Verification items for the finished model (mm, model axes). Round coordinates to 2 decimals unless told otherwise and drop trailing zeros. Write each loop counter-clockwise with the first axis right and the second up, starting at its lowest first coordinate (ties: lowest second). Pieces come first, ordered by that corner, then holes. Notation, with made-up numbers: M -33,82.5 L -10,82.5 A10 cw -10,86.5 Z; hole C 58.5,7.25 d5. An arc over 180 degrees is marked long. One line per question, with ' | ' between items. Start each with the question number.
Q1. Gauge pin test, flat ends, axial feed: pin 1 (4 mm diameter, centred on x = -49.5, z = -42.5, fed in from +Y); pin 2 (6.5 mm diameter, centred on x = -40, y = -33, fed in from -Z); pin 3 (3 mm diameter, centred on y = -12.5, z = -19, fed in from +X); pin 4 (8 mm diameter, centred on x = -29, y = -33.5, fed in from +Z). Record the tip position at first contact, or that the pin passes through.
Q2. Thickness scan on line 1 along Y through (x, z) = (-31, -17); line 2 along Y through (x, z) = (-51, -50); line 3 along X through (y, z) = (-3, -46.5). Record the ranges inside material, lowest first. Write a range as from..to.
Q3. Cross-section at B-B (z = -6). Record the boundary of the cut face in (x, y), then the cut area to 3 significant figures.
Q4. Cross-section at A-A (x = -56.5). Record the boundary of the cut face in (y, z), then the cut area to 3 significant figures.
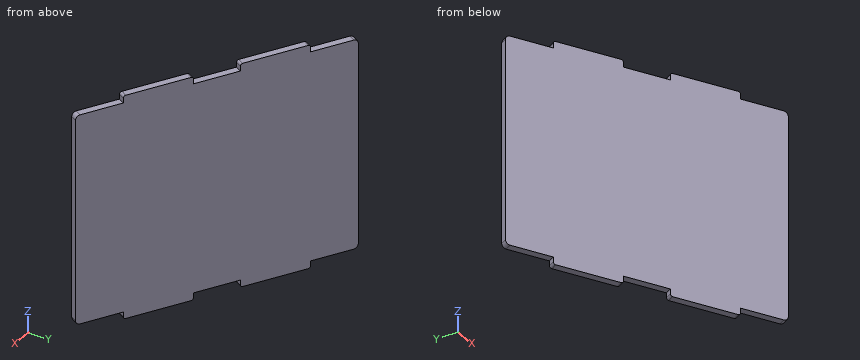
from build123d import *

# Parameters (mm, degrees)
EXTRUDE_THIN1_DEPTH = 100
CAVITY1_START       = -76.897726178
CAVITY1_OUTLINE_W   = 3.175
CAVITY1_OUTLINE_H   = 3.175
CAVITY1_DEPTH       = 20.486772374
CAVITY1_START_2     = 23.656985384
CAVITY1_2_OUTLINE_W = 3.175
CAVITY1_2_OUTLINE_H = 3.175
CAVITY1_2_DEPTH     = 20.486772374
CAVITY1_START_3     = -26.410953804
CAVITY1_3_OUTLINE_W = 3.175
CAVITY1_3_OUTLINE_H = 3.175
CAVITY1_3_DEPTH     = 20.067939188
FILLET1_R           = 2
FILLET2_R           = 1


# Read off the part's stored shape, not the designer's step: Cavity1
with BuildPart() as part:
    # Sketch1 → Extrude-Thin1 (new body)
    with BuildSketch(Plane.XY.offset(1.5875)):
        Polygon((-89.533643617, -1.281367376), (15.291356383, -61.802109344), (16.878856383, -59.052478687), (-87.946143617, 1.468263281), align=None)
    extrude(amount=-EXTRUDE_THIN1_DEPTH)

    # Cavity1 outline → Cavity1 (cut)
    with BuildSketch(Plane(origin=(0, 0, 0), x_dir=(0.5000000000000022, 0.8660254037844374, 0), z_dir=(0.8660254037844374, -0.5000000000000022, 0)).offset(CAVITY1_START)):
        with Locations((-44.289018508, -96.825)):
            Rectangle(CAVITY1_OUTLINE_W, CAVITY1_OUTLINE_H)
        with Locations((-44.289018508, 0)):
            Rectangle(CAVITY1_OUTLINE_W, CAVITY1_OUTLINE_H)
    extrude(amount=CAVITY1_DEPTH, mode=Mode.SUBTRACT)

    # Cavity1 2 outline → Cavity1 2 (cut)
    with BuildSketch(Plane(origin=(0, 0, 0), x_dir=(0.5000000000000022, 0.8660254037844374, 0), z_dir=(0.8660254037844374, -0.5000000000000022, 0)).offset(CAVITY1_START_2)):
        with Locations((-44.289018508, -96.825)):
            Rectangle(CAVITY1_2_OUTLINE_W, CAVITY1_2_OUTLINE_H)
        with Locations((-44.289018508, 0)):
            Rectangle(CAVITY1_2_OUTLINE_W, CAVITY1_2_OUTLINE_H)
    extrude(amount=CAVITY1_2_DEPTH, mode=Mode.SUBTRACT)

    # Cavity1 3 outline → Cavity1 3 (cut)
    with BuildSketch(Plane(origin=(0, 0, 0), x_dir=(0.5000000000000022, 0.8660254037844374, 0), z_dir=(0.8660254037844374, -0.5000000000000022, 0)).offset(CAVITY1_START_3)):
        with Locations((-44.289018508, -96.825)):
            Rectangle(CAVITY1_3_OUTLINE_W, CAVITY1_3_OUTLINE_H)
        with Locations((-44.289018508, 0)):
            Rectangle(CAVITY1_3_OUTLINE_W, CAVITY1_3_OUTLINE_H)
    extrude(amount=CAVITY1_3_DEPTH, mode=Mode.SUBTRACT)

    # Fillet1
    fillet1_edges = [part.edges().sort_by_distance(p)[0] for p in [
        (-88.739893617, 0.093447952, -1.5875),
        (16.085106383, -60.427294016, -1.5875),
        (16.085106383, -60.427294016, -95.2375),
        (-88.739893617, 0.093447952, -95.2375),
    ]]
    fillet(fillet1_edges, radius=FILLET1_R)

    # Fillet2
    fillet2_edges = [part.edges().sort_by_distance(p)[0] for p in [
        (-27.637721048, -35.183907829, -98.4125),
        (-1.656958934, -50.183907829, -98.4125),
        (-45.017066186, -25.149938235, -98.4125),
        (-70.9978283, -10.149938235, -98.4125),
        (-27.637721048, -35.183907829, 1.5875),
        (-45.017066186, -25.149938235, 1.5875),
        (-1.656958934, -50.183907829, 1.5875),
        (-70.9978283, -10.149938235, 1.5875),
    ]]
    fillet(fillet2_edges, radius=FILLET2_R)


solid = part.part
Determined:
1) pin 1: stops at y = -19.57 | pin 2: stops at z = -95.24 | pin 3: stops at x = -61.15 | pin 4: stops at z = 1.59
2) line 1: y = -35.08..-31.41 | line 2: y = -23.53..-19.86 | line 3: x = -86.56..-80.21
3) outline: M -89.53,-1.28 L 15.29,-61.8 L 16.88,-59.05 L -87.95,1.47 Z | area: 384 mm²
4) outline: M -20.35,-98.41 L -16.69,-98.41 L -16.69,1.59 L -20.35,1.59 Z | area: 367 mm²
